from build123d import *

# Parameters (mm, degrees)
SKETCH1_R               = 20
BOSS_EXTRUDE1_DEPTH     = 7.5
SKETCH4_R               = 5.125
CUT_EXTRUDE2_DEPTH      = 12.15
SKETCH5_R               = 2
CUT_EXTRUDE3_DEPTH      = 1
CUT_EXTRUDE3_DEPTH_BACK = 16
SKETCH2_R               = 2.025
CUT_EXTRUDE1_DEPTH      = 16
CIRPATTERN1_COUNT       = 4
SKETCH6_R               = 1.525
CUT_EXTRUDE4_DEPTH      = 21
CUT_EXTRUDE5_START      = -20
SKETCH7_R               = 3.25
CUT_EXTRUDE5_DEPTH      = 8
CUT_EXTRUDE11_START     = -6.5
CUT_EXTRUDE11_DEPTH     = 2.85
CIRPATTERN2_COUNT       = 2
CIRPATTERN2_ANGLE       = 135
CUT_EXTRUDE7_START      = 5.5
CUT_EXTRUDE7_DEPTH      = 3.75
CIRPATTERN3_COUNT       = 2
CUT_EXTRUDE12_START     = -16.0000001
SKETCH10_R              = 6
CUT_EXTRUDE12_DEPTH     = 17.0000002
CIRPATTERN4_COUNT       = 2
CIRPATTERN4_ANGLE       = 100


with BuildPart() as part:
    # Sketch1 → Boss-Extrude1 (new body, symmetric)
    with BuildSketch(Plane(origin=(0, 0, 0), x_dir=(1, 0, 0), z_dir=(0, 1, 0))):
        Circle(SKETCH1_R)
    extrude(amount=BOSS_EXTRUDE1_DEPTH, both=True)

    # Sketch4 → Cut-Extrude2 (cut)
    with BuildSketch(Plane.XZ.offset(7.5)):
        Circle(SKETCH4_R)
    extrude(amount=-CUT_EXTRUDE2_DEPTH, mode=Mode.SUBTRACT)

    # Sketch5 → Cut-Extrude3 (cut, two sides)
    with BuildSketch(Plane(origin=(0, 7.5, 0), x_dir=(1, 0, 0), z_dir=(0, 1, 0))) as cut_extrude3_sk:
        Circle(SKETCH5_R)
    extrude(amount=CUT_EXTRUDE3_DEPTH, mode=Mode.SUBTRACT)
    extrude(cut_extrude3_sk.sketch, amount=-CUT_EXTRUDE3_DEPTH_BACK, mode=Mode.SUBTRACT)

    # Sketch2 → Cut-Extrude1 (cut, through all)
    with BuildSketch(Plane(origin=(0, 7.5, 0), x_dir=(1, 0, 0), z_dir=(0, 1, 0))):
        with Locations((-13.807572802, 5.860966927)):
            Circle(SKETCH2_R)
    cut_extrude1 = extrude(amount=-CUT_EXTRUDE1_DEPTH, mode=Mode.SUBTRACT)

    # CirPattern1: Cut-Extrude1 ×4 about axis
    cirpattern1_axis = Axis((0, 0, 0), (0, 1, 0))
    for i in range(1, CIRPATTERN1_COUNT):
        add(cut_extrude1.rotate(cirpattern1_axis, i * 360 / CIRPATTERN1_COUNT), mode=Mode.SUBTRACT)

    # Sketch6 → Cut-Extrude4 (cut, through all)
    with BuildSketch(Plane.XY):
        with Locations((0, -1.35)):
            Circle(SKETCH6_R)
    cut_extrude4 = extrude(amount=-CUT_EXTRUDE4_DEPTH, mode=Mode.SUBTRACT)

    # Sketch7 → Cut-Extrude5 (cut)
    with BuildSketch(Plane.XY.offset(CUT_EXTRUDE5_START)):
        with Locations((0, -1.35)):
            Circle(SKETCH7_R)
    cut_extrude5 = extrude(amount=CUT_EXTRUDE5_DEPTH, mode=Mode.SUBTRACT)

    # Sketch9 → Cut-Extrude11 (cut)
    with BuildSketch(Plane.XY.offset(CUT_EXTRUDE11_START)):
        Polygon((3.125, -3.154219591), (3.125, 0.454219591), (0, 2.258439182), (-3.125, 0.454219591), (-3.125, -3.154219591), (-3.125, -7.670640979), (3.125, -7.670640979), align=None)
    cut_extrude11 = extrude(amount=-CUT_EXTRUDE11_DEPTH, mode=Mode.SUBTRACT)

    # CirPattern2: Cut-Extrude4, Cut-Extrude5, Cut-Extrude11 ×2 about axis
    cirpattern2_axis = Axis((0, 0, 0), (0, 1, 0))
    for i in range(1, CIRPATTERN2_COUNT):
        add(cut_extrude4.rotate(cirpattern2_axis, i * CIRPATTERN2_ANGLE / (CIRPATTERN2_COUNT - 1)), mode=Mode.SUBTRACT)
        add(cut_extrude5.rotate(cirpattern2_axis, i * CIRPATTERN2_ANGLE / (CIRPATTERN2_COUNT - 1)), mode=Mode.SUBTRACT)
        add(cut_extrude11.rotate(cirpattern2_axis, i * CIRPATTERN2_ANGLE / (CIRPATTERN2_COUNT - 1)), mode=Mode.SUBTRACT)

    # Sketch8 → Cut-Extrude7 (cut)
    with BuildSketch(Plane(origin=(0, 0, 0), x_dir=(1, 0, 0), z_dir=(0, 1, 0)).offset(CUT_EXTRUDE7_START)):
        Polygon((-9.423079571, 3.999859969), (-10.003560281, 8.727495969), (-14.388053512, 10.588602927), (-19.566381078, 12.786672569), (-22.789912888, 5.192507528), (-17.611585322, 2.994437886), (-13.227092091, 1.133330928), align=None)
    cut_extrude7 = extrude(amount=-CUT_EXTRUDE7_DEPTH, mode=Mode.SUBTRACT)

    # CirPattern3: Cut-Extrude7 ×2 about axis
    cirpattern3_axis = Axis((0, 0, 0), (0, 1, 0))
    for i in range(1, CIRPATTERN3_COUNT):
        add(cut_extrude7.rotate(cirpattern3_axis, i * 360 / CIRPATTERN3_COUNT), mode=Mode.SUBTRACT)

    # Sketch10 → Cut-Extrude12 (cut)
    with BuildSketch(Plane(origin=(0, 7.5, 0), x_dir=(1, 0, 0), z_dir=(0, 1, 0)).offset(CUT_EXTRUDE12_START)):
        with Locations((3.654646309, -11.95380945)):
            Circle(SKETCH10_R)
    cut_extrude12 = extrude(amount=CUT_EXTRUDE12_DEPTH, mode=Mode.SUBTRACT)

    # CirPattern4: Cut-Extrude12 ×2 about axis
    cirpattern4_axis = Axis((0, 7.5, 0), (0, 1, 0))
    for i in range(1, CIRPATTERN4_COUNT):
        add(cut_extrude12.rotate(cirpattern4_axis, i * CIRPATTERN4_ANGLE / (CIRPATTERN4_COUNT - 1)), mode=Mode.SUBTRACT)


solid = part.part
The model under review builds one solid part; all positions refer to its coordinate system, in mm. A direction names the side the tool comes from. Round coordinates to 2 decimals unless told otherwise and drop trailing zeros. Loops run counter-clockwise (first coordinate to the right, second up) from the corner with the lowest first, then second, coordinate; pieces in that order, holes last. Notation, with made-up numbers: M 43.25,-15 L 65.25,-15 A21 cw 65.25,14 Z; hole C 61,33 d3. An arc over 180 degrees is marked long. Answer as CSV lines item,"result".
1. Insertion check: pin 1 Ø3.5 at (x, y) = (0, -1.35) entering from -Z; pin 2 Ø1.8 at (x, y) = (0, -1.35) entering from -Z; pin 3 Ø2 at (y, z) = (3.5, -4.5) entering from -X; pin 4 Ø2.5 at (x, z) = (0, 0) entering from +Y. Each pin has a flat end and moves straight along its axis. Give the tip position at first contact, or say it passes through.
Outcome:
pin 1,"stops at z = -12"
pin 2,"stops at z = 5.05"
pin 3,"stops at x = -19.69"
pin 4,"passes through"
2. For faces 1 (the face through (-9.71, 3.65, -6.33)), 2 (the face through (1, -3, -12)), 3 (the face through (-6.581, -3.637, 6.642)), list the 3-axis set-ups (+Z, -Z, +X, -X, +Y, -Y) from which the entire face can be reached by the end or side of a thin tool; tool diameter is ignored.
Outcome:
face 1,"-X"
face 2,"-Z"
face 3,"-Y"
3. We need section A-A (z = -14). Give the boundary of the cut face in (x, y), plus the area to 3 significant figures.
Outcome:
outline,"M -14.28,-7.5 L 3.85,-7.5 L 3.85,7.5 L -14.28,7.5 Z; M 7.88,-7.5 L 14.28,-7.5 L 14.28,7.5 L 7.88,7.5 Z; hole C 0,-1.35 d6.5"
area,"335 mm2"
4. We need section C-C (y = -6). Count the separate pieces of the cut face and the enclosed holes in it, plus the area to 3 significant figures.
Outcome:
separate pieces,"1"
enclosed holes,"9"
area,"861 mm2"
5. Draft analysis for pull direction Z (two halves, no side actions). For faces 4 (the face through (-5, -7.5, -5)), 5 (the face through (19.076, 0.105, -6.007)), 6 (the face through (1.584, 1.344, -7.905)), state which applies: pulls with the +Z half, pulls with the -Z half, needs draft (parallel to the pull), parting line crosses it, or undercut.
Outcome:
face 4,"needs draft"
face 5,"parting line crosses it"
face 6,"undercut"
6. To check wall thickness, follow L1, parallel to Z at x = 6, y = 3.75; L2, parallel to Z at x = -3, y = -6.25; L3, parallel to Y at x = -15, z = -10. State the ranges of each line that lie inside material, in increasing order. Write a range as [from, to].
Outcome:
L1,"z = [-19.08, -15.83], [-11.79, -8.77], [-2.58, 6.43], [17.48, 19.08]"
L2,"z = [-19.77, -9.35], [-6.5, -4.16], [4.16, 6.19], [7.42, 19.77]"
L3,"y = [-7.5, 1.75], [5.5, 7.5]"
7. We need section B-B (x = 11). Give the boundary of the cut face in (y, z), plus the area to 3 significant figures.
Outcome:
outline,"M -7.5,-16.7 L 7.5,-16.7 L 7.5,-11.67 L -7.5,-11.67 Z; M -7.5,0.32 L 7.5,0.32 L 7.5,16.7 L -7.5,16.7 Z; hole M 1.75,2.81 L 5.5,2.81 L 5.5,9.15 L 1.75,9.15 Z"
area,"297 mm2"
